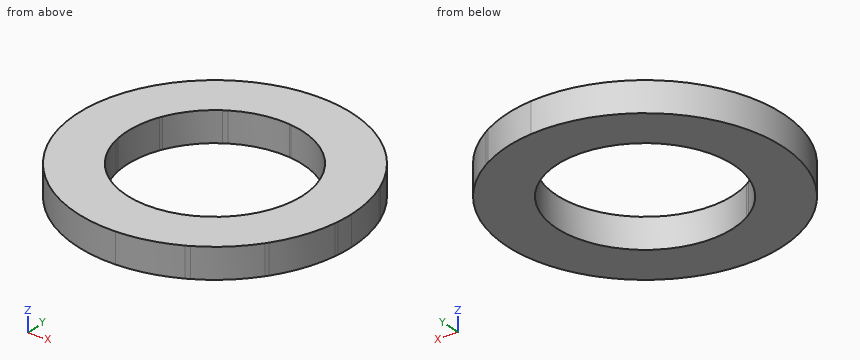
```python
from build123d import *

# Parameters (mm, degrees)
F1_DEPTH = 5.1


with BuildPart() as f1:
    # F0 (on Top) → F1 (new body)
    with BuildSketch(Plane.XY):
        with BuildLine():
            ThreePointArc((23.0623797864, -2.752888696), (23.1851344055, -1.378876421), (23.2261007831, 0))
            ThreePointArc((23.2261007831, 0), (22.8721340644, 4.039460475), (21.8210228424, 7.9557978667))
            ThreePointArc((21.8210228424, 7.9557978667), (21.7129320627, 8.2462317956), (21.600975855, 8.5351976954))
            ThreePointArc((21.600975855, 8.5351976954), (17.6168585154, 15.135985387), (11.6914938176, 20.0688995687))
            ThreePointArc((11.6914938176, 20.0688995687), (11.3296656288, 20.2753652082), (10.9641925592, 20.4753080346))
            ThreePointArc((10.9641925592, 20.4753080346), (6.4344525637, 22.3170243938), (1.6195142321, 23.1695690775))
            ThreePointArc((1.6195142321, 23.1695690775), (-23.2232414227, 0.3644384862), (0.891703377, -23.2089772001))
            ThreePointArc((0.891703377, -23.2089772001), (5.9586225424, -22.4487544194), (10.7355743028, -20.5960967655))
            ThreePointArc((10.7355743028, -20.5960967655), (11.0730407687, -20.4166482489), (11.4075086171, -20.231670834))
            ThreePointArc((11.4075086171, -20.231670834), (15.509940512, -17.2885367484), (18.8794446221, -13.5284266767))
            ThreePointArc((18.8794446221, -13.5284266767), (19.0526450726, -13.283390882), (19.2226654093, -13.0361379307))
            ThreePointArc((19.2226654093, -13.0361379307), (21.6572092153, -8.3914865543), (22.9877271358, -3.3190599146))
            ThreePointArc((22.9877271358, -3.3190599146), (23.0267936185, -3.0362037542), (23.0623797864, -2.752888696))
        make_face()
        with BuildLine():
            ThreePointArc((-7.6265143045, 12.7618767873), (-3.3183069466, 14.491999813), (1.3134897969, 14.8089150219))
            ThreePointArc((1.3134897969, 14.8089150219), (1.4665804544, 14.7945382268), (1.6195142321, 14.7785788635))
            ThreePointArc((1.6195142321, 14.7785788635), (11.0703798721, 9.9235028624), (14.8670514754, 0))
            ThreePointArc((14.8670514754, 0), (7.4772282889, -12.8499134895), (-7.3458637029, -12.9254596062))
            ThreePointArc((-7.3458637029, -12.9254596062), (-7.689867558, -12.7238027536), (-8.0283394714, -12.5129926438))
            ThreePointArc((-8.0283394714, -12.5129926438), (-9.5257186584, -11.4144602856), (-10.874459487, -10.1378178341))
            ThreePointArc((-10.874459487, -10.1378178341), (-11.0561755007, -9.9393260772), (-11.2342689854, -9.7375777243))
            ThreePointArc((-11.2342689854, -9.7375777243), (-13.3519365266, -6.5387315713), (-14.5805712978, -2.9045068776))
            ThreePointArc((-14.5805712978, -2.9045068776), (-14.6272984034, -2.6592030743), (-14.6698988149, -2.4131490494))
            ThreePointArc((-14.6698988149, -2.4131490494), (-14.7754620576, 1.6477076674), (-13.7779120757, 5.5855490693))
            ThreePointArc((-13.7779120757, 5.5855490693), (-13.6764347777, 5.8296098793), (-13.570634607, 6.0718280554))
            ThreePointArc((-13.570634607, 6.0718280554), (-11.3456382043, 9.6075862374), (-8.2248041845, 12.3847412448))
            ThreePointArc((-8.2248041845, 12.3847412448), (-7.9279021351, 12.57686715), (-7.6265143045, 12.7618767873))
        make_face(mode=Mode.SUBTRACT)
    extrude(amount=F1_DEPTH)


solid = f1.part
```
Work out the finished part from the listing and answer in its coordinate system (mm). Give positions to 0.01 mm unless a question says otherwise; leave off trailing zeros. Order: outer loops, then holes, each group sorted by start corner. A loop starts at its lowest first (then second) coordinate and runs counter-clockwise, first axis right, second up. Notation, with made-up numbers: (63.25, 39) - (81.25, 39) arc R24 cw to (81.25, 76) - close; hole circle Ø10 at (-1.75, -8.5). An arc over 180 degrees is marked (long way). One line per item, written item: value. Start each with the question number.
1. Consider line 1 (Y direction, x = 0, z = 2.5); line 2 (X direction, y = -4, z = 3.6). Determine where each line is inside the solid, lowest interval first.
2. Each of these flat-tipped pins is pushed along its axis until it touches: pin 1 Ø1.5 at (y, z) = (5, 1.5) entering from +X; pin 2 Ø1.5 at (y, z) = (-7.5, 0.5) entering from +X; pin 3 Ø1.5 at (y, z) = (-16, 3.5) entering from +X. Where does it stop, or does it pass through?
3. Section A-A, the plane x = 0 is taken. Write down the section's boundary in (y, z).
4. Section B-B, the plane y = 2.5 is taken. Write down the section's boundary in (x, z), then the cut area to 3 significant figures.
5. Section C-C, the plane z = 3.55 is taken. Write down the section's boundary in (x, y).
Filled sheet:
1. line 1: -23.23 to -14.87, 14.87 to 23.23
1. line 2: -22.88 to -14.32, 14.32 to 22.88
2. pin 1: x = 22.83
2. pin 2: x = 22.22
2. pin 3: x = 17.52
3. outline: (-23.23, 0) - (-14.87, 0) - (-14.87, 5.1) - (-23.23, 5.1) - close; (14.87, 0) - (23.23, 0) - (23.23, 5.1) - (14.87, 5.1) - close
4. outline: (-23.09, 0) - (-14.66, 0) - (-14.66, 5.1) - (-23.09, 5.1) - close; (14.66, 0) - (23.09, 0) - (23.09, 5.1) - (14.66, 5.1) - close
4. area: 86.0 mm²
5. outline: circle Ø46.45 at (0, 0); hole circle Ø29.73 at (0, 0)
